from build123d import *

# Parameters (mm, degrees)
F1_DEPTH = 50.1
F3_D     = 9
F5_D     = 9
F5_DEPTH = 35
F5_TIP   = 2.7038727856


with BuildPart() as f1:
    # F0 (on Front) → F1 (new body)
    with BuildSketch(Plane.XZ):
        with BuildLine():
            Line((0, 20.1881089388), (0, 38.1235034296))
            Line((0, 38.1235034296), (-20, 38.1235034296))
            Line((-20, 38.1235034296), (-20, 7.6235034296))
            Line((-20, 7.6235034296), (-12.4, -1.9764965704))
            Line((-12.4, -1.9764965704), (-12.4, -36.0764965704))
            Line((-12.4, -36.0764965704), (-2.4, -36.0764965704))
            Line((-2.4, -36.0764965704), (-2.4, 3.9235034296))
            ThreePointArc((-2.4, 3.9235034296), (-9.9117323022, 13.3413066234), (0, 20.1881089388))
        make_face()
    extrude(amount=-F1_DEPTH)

    # F3 (through all)
    with Locations(Plane.YZ):
        with Locations((13.5, 30.1235034296), (36.6, 30.1235034296)):
            Hole(F3_D / 2)

    # F5
    with Locations(Plane.XY.offset(38.1235034296)):
        with Locations((-10, 26.6)):
            Hole(F5_D / 2, depth=F5_DEPTH)
            with Locations((0, 0, -(F5_DEPTH + F5_TIP / 2))):  # 118° drill point
                Cone(0, F5_D / 2, F5_TIP, mode=Mode.SUBTRACT)


solid = f1.part
Can you work these out from the model? Positions are in its coordinate system, mm. A direction names the side the tool comes from. Coordinates: 2 decimals unless noted, no trailing zeros. Loops run counter-clockwise (first coordinate to the right, second up) from the corner with the lowest first, then second, coordinate; pieces in that order, holes last. Notation, with made-up numbers: M -25.5,57 L 4.5,57 A24 cw 4.5,88 Z; hole C -34,-3 d10. An arc over 180 degrees is marked long. Return JSON: item names as keys, results as strings. Group by question number.
Item 1: If I drill on L1, parallel to Y at x = -10, z = 15.5; L2, parallel to Z at x = -4, y = 36.6; L3, parallel to Z at x = -7, y = 13.5, over which ranges is the centre line in solid material (lowest first)? Write a range as from..to.
Item 2: Imagine slicing it at B-B (y = 44). Please give me the cut outline in (x, z), and give its area (3 significant figures).
Item 3: I'm going to push flat-ended pins straight in: pin 1 Ø10 at (y, z) = (24, -25) entering from -X; pin 2 Ø5.5 at (y, z) = (13.5, 30.12) entering from -X; pin 3 Ø3 at (y, z) = (13, 1) entering from +X; pin 4 Ø5 at (y, z) = (24.5, 14.5) entering from +X. Where does each tip first touch, or does it pass through?
Item 4: Imagine slicing it at A-A (y = 13.5). Please give me the cut outline in (x, z), and give its area (3 significant figures).
Item 5: On a 3-axis mill with a long thin cutter (end or side, diameter ignored), from which of +Z, -Z, +X, -X, +Y, -Y can I reach the whole of each face in a straight line? I mean faces 4 (the flat face through (-2.4, 25, -16)), 5 (the flat face through (-12.4, 25, -19)), 6 (the cylindrical face through (-14.292, 27.952, 20.379)). Say none if no direction works.
Item 6: Imagine slicing it at C-C (z = -30.5). Please give me the cut outline in (x, y).
Item 7: Thinking about a two-plate mould opening in Y: for faces 1 (the flat face through (0, 25, 29)), 2 (the cylindrical face through (-10.14, 14.48, 25.73)), 3 (the flat face through (-10, 0, 10)), which applies, released by +Y, released by -Y, zero draft, split by the parting line, or undercut?
Item 8: Imagine slicing it at D-D (x = -11.25). Give the number of separate pieces and of enclosed holes in the cut face, and give its area (3 significant figures).
Verdict:
{
 "1": {"L1": "y = 0..22.1, 31.1..50.1", "L2": "z = -36.08..4.21, 20.07..25.62, 34.62..38.12", "L3": "z = -36.08..5.78, 18.5..25.62, 34.62..38.12"},
 "2": {"outline": "M -20,7.62 L -12.4,-1.98 L -12.4,-36.08 L -2.4,-36.08 L -2.4,3.92 A8.24 cw long 0,20.19 L 0,38.12 L -20,38.12 Z", "area": "957 mm^2"},
 "3": {"pin 1": "stops at x = -12.4", "pin 2": "passes through", "pin 3": "stops at x = -2.4", "pin 4": "stops at x = -9.35"},
 "4": {"outline": "M -20,7.62 L -12.4,-1.98 L -12.4,-36.08 L -2.4,-36.08 L -2.4,3.92 A8.24 cw long 0,20.19 L 0,25.62 L -20,25.62 Z; M -20,34.62 L 0,34.62 L 0,38.12 L -20,38.12 Z", "area": "777 mm^2"},
 "5": {"face 4": "-Z, +X, +Y, -Y", "face 5": "-Z, -X, +Y, -Y", "face 6": "+Z"},
 "6": {"outline": "M -12.4,0 L -2.4,0 L -2.4,50.1 L -12.4,50.1 Z"},
 "7": {"face 1": "zero draft", "face 2": "undercut", "face 3": "released by -Y"},
 "8": {"separate pieces": "1", "enclosed holes": "2", "area": "3,280 mm^2"}
}
